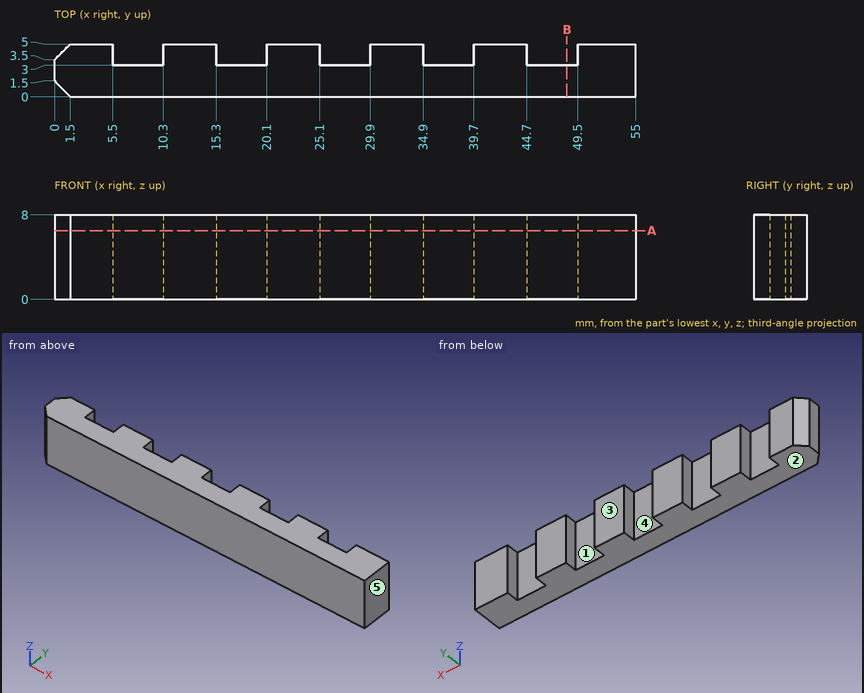
Print and shaded views of the part. All mm, measured from the part's lowest x, y and z. A direction names the side the tool comes from. Round coordinates to 2 decimals unless told otherwise and drop trailing zeros. Loops run counter-clockwise (first coordinate to the right, second up) from the corner with the lowest first, then second, coordinate; pieces in that order, holes last. Notation, with made-up numbers: M 59,29 L 80,29 A22 ccw 80,65 Z; hole C 50,51.25 d7. An arc over 180 degrees is marked long. One line per question, with ' | ' between items.
1) Mould opens along X. For the marked faces 3, 4 and 5 say: +X half, -X half, draft (parallel to the pull), parting line (faces both ways), or undercut.
Solved:
face 3: draft | face 4: undercut | face 5: +X half
2) Flat gauge pins, fed straight in: pin 1 (2.5 mm diameter, centred on x = 37.5, z = 2.5, fed in from +Y); pin 2 (0.6 mm diameter, centred on y = 4.5, z = 3.5, fed in from -X). Where does each tip first touch, or does it go through?
Solved:
pin 1: stops at y = 3 | pin 2: stops at x = 0.7
3) Band-saw the part on B-B (x = 48.5). Give the cut face in (y, z).
Solved:
outline: M 0,0 L 3,0 L 3,8 L 0,8 Z
4) 3-axis set-ups, long thin cutter, end or side, ignore diameter. For the marked faces 1 and 2: which of +Z, -Z, +X, -X, +Y, -Y reach the whole face in a straight line?
Solved:
face 1: +Z, -Z, +Y | face 2: -Z, +X, -X, +Y, -Y
5) Band-saw the part on A-A (z = 6.5). Give the cut face in (x, y), then the cut area to 3 significant figures.
Solved:
outline: M 0,1.5 L 1.5,0 L 55,0 L 55,5 L 49.5,5 L 49.5,3 L 44.7,3 L 44.7,5 L 39.7,5 L 39.7,3 L 34.9,3 L 34.9,5 L 29.9,5 L 29.9,3 L 25.1,3 L 25.1,5 L 20.1,5 L 20.1,3 L 15.3,3 L 15.3,5 L 10.3,5 L 10.3,3 L 5.5,3 L 5.5,5 L 1.5,5 L 0,3.5 Z | area: 225 mm²
6) Drill centre lines: line 1 along X through (y, z) = (3.1, 2.25); line 2 along Y through (x, z) = (9, 6.5); line 3 along X through (y, z) = (4.55, 1.5). Where is each one in solid material? Low to high.
Solved:
line 1: x = 0 to 5.5, 10.3 to 15.3, 20.1 to 25.1, 29.9 to 34.9, 39.7 to 44.7, 49.5 to 55 | line 2: y = 0 to 3 | line 3: x = 1.05 to 5.5, 10.3 to 15.3, 20.1 to 25.1, 29.9 to 34.9, 39.7 to 44.7, 49.5 to 55
